Work out the finished part from the listing and answer in its coordinate system (mm). Give positions to 0.01 mm unless a question says otherwise; leave off trailing zeros. Order: outer loops, then holes, each group sorted by start corner. A loop starts at its lowest first (then second) coordinate and runs counter-clockwise, first axis right, second up. Notation, with made-up numbers: M -25.5,-28 L -17.5,-28 A17 cw -17.5,0 Z; hole C 41.5,-26.75 d1. An arc over 180 degrees is marked long. One line per item, written item: value.
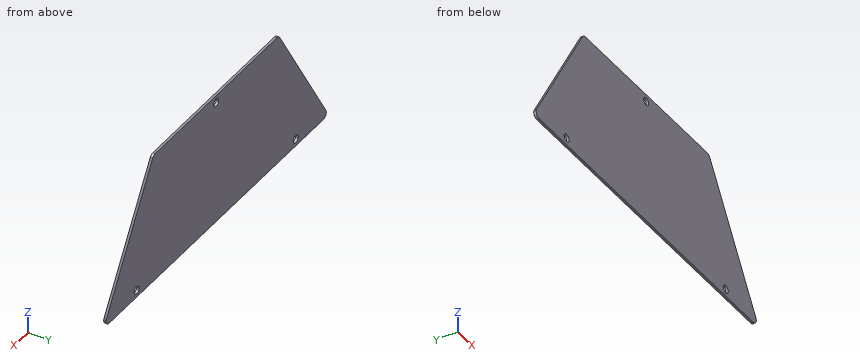
Autodesk Inventor part; units mm, degrees
ref_plane "YZ Plane" through (0, 0, 0) normal (1, 0, 0) x (0, 1, 0)
ref_plane "XZ Plane" through (0, 0, 0) normal (0, 1, 0) x (-1, 0, 0)
ref_plane "XY Plane" through (0, 0, 0) normal (0, 0, 1) x (1, 0, 0)
sketch "Sketch1" plane through (0, 0, 0) normal (0, 1, 0) x (-1, 0, 0)
  circle A0 centre (-37, 5.818) radius 1.6079
  circle A1 centre (13.7917, 54.8205) radius 1.6079
  line L0 (13.7917, 57.8205) -> (-25.0536, 57.8205)
  line L1 (-26.7857, 56.8205) -> (-56.232, 5.818)
  line L2 (64.5833, 2.818) -> (-37, 2.818)
  line L3 (-54.5, 2.818) -> (-37, 2.818)
  line L4 (13.7917, 57.8205) -> (52.637, 57.8205)
  line L5 (54.369, 56.8205) -> (83.8153, 5.818)
  line L6 (82.0833, 2.818) -> (64.5833, 2.818)
  circle A2 centre (64.5833, 5.818) radius 1.6079
  arc A3 (82.0833, 2.818) -> (83.8153, 5.818) centre (82.0833, 4.818) ccw
  arc A4 (-56.232, 5.818) -> (-54.5, 2.818) centre (-54.5, 4.818) ccw
  arc A5 (-25.0536, 57.8205) -> (-26.7857, 56.8205) centre (-25.0536, 55.8205) ccw
  arc A6 (54.369, 56.8205) -> (52.637, 57.8205) centre (52.637, 55.8205) ccw
  dimension "d13" = 2
  dimension "d14" = 2
extrude "Extrusion1" add sketch "Sketch1" along normal blind 1
properties part number "Veroboard"
(1) Section B-B, the plane x = 37 is taken. Give the vertices of the cut face in (y, z), then the cut area to 3 significant figures.
Findings:
outline: M 0,2.82 L 1,2.82 L 1,4.21 L 0,4.21 Z; M 0,7.43 L 1,7.43 L 1,39.13 L 0,39.13 Z
area: 33.1 mm^2
(2) Section A-A, the plane y = 0.6 is taken. Give the vertices of the cut face in (x, z).
Findings:
outline: M -83.82,5.82 A2 ccw -82.08,2.82 L 54.5,2.82 A2 ccw 56.23,5.82 L 26.79,56.82 A2 ccw 25.05,57.82 L -52.64,57.82 A2 ccw -54.37,56.82 Z; hole C -64.58,5.82 d3.22; hole C -13.79,54.82 d3.22; hole C 37,5.82 d3.22
(3) Section D-D, the plane z = 38.5 is taken. Give the vertices of the cut face in (x, y), then the cut area to 3 significant figures.
Findings:
outline: M -64.95,0 L 37.36,0 L 37.36,1 L -64.95,1 Z
area: 102 mm^2
(4) Section C-C, the plane z = 9.5 is taken. Give the vertices of the cut face in (x, y).
Findings:
outline: M -81.69,0 L 54.11,0 L 54.11,1 L -81.69,1 Z
(5) Find the intervals of material crossed by probe 1 along Z at (x, y) = (37, 0.7); probe 2 along X at (y, z) = (0.1, 12); probe 3 along X at (y, z) = (0.2, 49), in increasing order. Write a range as from..to.
Findings:
probe 1: z = 2.82..4.21, 7.43..39.13
probe 2: x = -80.25..52.66
probe 3: x = -58.88..31.3
